Build history of the part. All positions in model axes, mm. A direction names the side the tool comes from. Give positions to 0.01 mm unless a question says otherwise; leave off trailing zeros. Write each loop counter-clockwise with the first axis right and the second up, starting at its lowest first coordinate (ties: lowest second). Pieces come first, ordered by that corner, then holes. Notation, with made-up numbers: M -19,42 L -1,42 A13 ccw -1,49 Z; hole C 88.25,-2 d9. An arc over 180 degrees is marked long. One line per item, written item: value. Start each with the question number.
from build123d import *

# Parameters (mm, degrees)
F1_DEPTH = 12.7
F2_W     = 12.7
F2_H     = 76.2
F3_DEPTH = 50.8


with BuildPart() as f1:
    # F0 (on Right) → F1 (new body)
    with BuildSketch(Plane.YZ):
        Polygon((-44.519397, -30.93571), (-44.519397, -56.33571), (-31.819397, -56.33571), (-19.119397, -56.33571), (-19.119397, 19.86429), (-69.919397, 19.86429), (-69.919397, -5.53571), (-44.519397, -5.53571), (-44.519397, -18.23571), (-57.219397, -18.23571), (-57.219397, -30.93571), align=None)
    extrude(amount=F1_DEPTH)

    # F2 (on face) → F3 (join)
    with BuildSketch(Plane.YZ.offset(12.7)):
        with Locations((-25.469397, -18.23571)):
            Rectangle(F2_W, F2_H)
    extrude(amount=F3_DEPTH)


solid = f1.part
1) Mould opens along Z. For faces 4 (the face through (24, -26, -56.336)), 5 (the face through (17, -28, 19.864)), 6 (the face through (63.5, -26, -18)), 7 (the face through (6, -51, -18.236)) say: released by +Z, released by -Z, zero draft, split by the parting line, or undercut.
2) Band-saw the part on D-D (y = -40.5). List the corners of the cut face in (x, z).
3) Band-saw the part on B-B (x = 9.5). List the corners of the cut face in (y, z).
4) Band-saw the part on A-A (y = -53.5). List the corners of the cut face in (x, z).
5) Drop flat-ended pins along their axis: P1, Ø1.5, axis at y = -48, z = -28.5, coming from the -X side; P2, Ø10, axis at x = 9.5, y = -51.5, coming from the -Z side; P3, Ø14, axis at x = 8.5, z = -22.5, coming from the -Y side; P4, Ø4, axis at y = -37.5, z = -8, coming from the +X side. Give the stop position or say it passes through.
6) Tool access for faces 1 (the face through (6, -57, -5.536)), 2 (the face through (6, -51, -30.936)), 3 (the face through (12.7, -43, -9)): list every direction of +Z, -Z, +X, -X, +Y, -Y with a clear straight run to the whole face (end or side of a thin tool).
7) Band-saw the part on C-C (z = -7). List the corners of the cut face in (x, y), then the cut area to 3 significant figures.
8) Probe line 1 along Z through (x, y) = (7, -49.5); line 2 along X through (y, z) = (-37, -43); line 3 along Y through (x, z) = (50, -12.5). List the from-to ranges inside material, lowest first. Write a range as from..to.
Model answer:
1. face 4: released by -Z
1. face 5: released by +Z
1. face 6: zero draft
1. face 7: undercut
2. outline: M 0,-56.34 L 12.7,-56.34 L 12.7,19.86 L 0,19.86 Z
3. outline: M -69.92,-5.54 L -44.52,-5.54 L -44.52,-18.24 L -57.22,-18.24 L -57.22,-30.94 L -44.52,-30.94 L -44.52,-56.34 L -19.12,-56.34 L -19.12,19.86 L -69.92,19.86 Z
4. outline: M 0,-30.94 L 12.7,-30.94 L 12.7,-18.24 L 0,-18.24 Z; M 0,-5.54 L 12.7,-5.54 L 12.7,19.86 L 0,19.86 Z
5. P1: stops at x = 0
5. P2: stops at z = -30.94
5. P3: stops at y = -57.22
5. P4: stops at x = 12.7
6. face 1: +X, -X, -Y
6. face 2: -Z, +X, -X, -Y
6. face 3: +Z, -Z, +X, -Y
7. outline: M 0,-44.52 L 12.7,-44.52 L 12.7,-31.82 L 63.5,-31.82 L 63.5,-19.12 L 0,-19.12 Z
7. area: 968 mm²
8. line 1: z = -30.94..-18.24, -5.54..19.86
8. line 2: x = 0..12.7
8. line 3: y = -31.82..-19.12
